Geometry: final body of the model. Coordinates: model frame, mm. Face numbers are marked on the shaded views. Coordinates: 2 decimals unless noted, no trailing zeros. Put each result on its own line as item: value.
```python
from build123d import *

# Parameters (mm, degrees)
CROQUIS1_R                  = 16.5
CROQUIS1_R_2                = 3.75
CROQUIS1_R_3                = 1.5
SALIENTE_EXTRUIR1_DEPTH     = 5
CROQUIS2_R                  = 5.5
CORTAR_EXTRUIR1_DEPTH       = 2
CORTAR_EXTRUIR2_START       = -5
CROQUIS4_R                  = 3
CORTAR_EXTRUIR2_DEPTH       = 2.5
CROQUIS6_R                  = 1.5
SALIENTE_EXTRUIR3_DEPTH     = 5
SALIENTE_EXTRUIR4_START     = -5
SALIENTE_EXTRUIR4_DEPTH     = 5
CORTAR_EXTRUIR3_START       = -5
CORTAR_EXTRUIR3_OUTLINE_R   = 1.5
CORTAR_EXTRUIR3_OUTLINE_R_2 = 3.75
CORTAR_EXTRUIR3_DEPTH       = 5


# Read off the part's stored shape, not the designer's step: Saliente-Extruir4, Cortar-Extruir3
with BuildPart() as part:
    # Croquis1 → Saliente-Extruir1 (new body)
    with BuildSketch(Plane(origin=(0, 0, 0), x_dir=(1, 0, 0), z_dir=(0, 1, 0))):
        with Locations(Location((0, 0, 0), (0, 0, 270))):
            Circle(CROQUIS1_R)
        with Locations(Location((0, 0, 0), (0, 0, 270))):
            Circle(CROQUIS1_R_2, mode=Mode.SUBTRACT)
        with Locations(Location((10, 0, 0), (0, 0, 270))):
            Circle(CROQUIS1_R_3, mode=Mode.SUBTRACT)
        with Locations(Location((0, -10, 0), (0, 0, 270))):
            Circle(CROQUIS1_R_3, mode=Mode.SUBTRACT)
        with Locations(Location((-10, 0, 0), (0, 0, 270))):
            Circle(CROQUIS1_R_3, mode=Mode.SUBTRACT)
        with Locations(Location((0, 10, 0), (0, 0, 270))):
            Circle(CROQUIS1_R_3, mode=Mode.SUBTRACT)
    extrude(amount=SALIENTE_EXTRUIR1_DEPTH)

    # Croquis2 → Cortar-Extruir1 (cut)
    with BuildSketch(Plane(origin=(0, 5, 0), x_dir=(1, 0, 0), z_dir=(0, 1, 0))):
        with Locations(Location((0, 0, 0), (0, 0, 270))):
            Circle(CROQUIS2_R)
    extrude(amount=-CORTAR_EXTRUIR1_DEPTH, mode=Mode.SUBTRACT)

    # Croquis4 → Cortar-Extruir2 (cut)
    with BuildSketch(Plane(origin=(0, 5, 0), x_dir=(1, 0, 0), z_dir=(0, 1, 0)).offset(CORTAR_EXTRUIR2_START)):
        with Locations(Location((10, 0, 0), (0, 0, 270))):
            Circle(CROQUIS4_R)
        with Locations(Location((-10, 0, 0), (0, 0, 270))):
            Circle(CROQUIS4_R)
        with Locations(Location((0, 10, 0), (0, 0, 270))):
            Circle(CROQUIS4_R)
    extrude(amount=CORTAR_EXTRUIR2_DEPTH, mode=Mode.SUBTRACT)

    # Croquis6 → Saliente-Extruir3 (add)
    with BuildSketch(Plane(origin=(0, 5, 0), x_dir=(1, 0, 0), z_dir=(0, 1, 0))):
        with BuildLine():
            Line((-16.499999253, -0.004966275), (0, -15.162135144))
            Line((0, -15.162135144), (16.499999253, -0.004966275))
            add(Edge.make_bspline(
                [(16.499999253, -0.004966275), (14.789720677, -16.601874141), (14.779811161, -16.438973164), (14.200732618, -20.551745369), (13.635520661, -22.485602375), (15.733267293, -30.419610193), (11.37636727, -34.073606125), (1.56418736, -36.497980996), (2.416281914, -27.975905143), (1.888822796, -23.5), (0, -23.5)],
                knots=[0, 0, 0, 0, 0.196162037, 0.24321543, 0.470533934, 0.661030556, 0.708413553, 0.918147195, 0.949927511, 1, 1, 1, 1], degree=3))
            add(Edge.make_bspline(
                [(-16.499999253, -0.004966275), (-14.789720677, -16.601874141), (-14.779811161, -16.438973164), (-14.200732618, -20.551745369), (-13.635520661, -22.485602375), (-15.733267293, -30.419610193), (-11.37636727, -34.073606125), (-1.56418736, -36.497980996), (-2.416281914, -27.975905143), (-1.888822796, -23.5), (0, -23.5)],
                knots=[0, 0, 0, 0, 0.196162037, 0.24321543, 0.470533934, 0.661030556, 0.708413553, 0.918147195, 0.949927511, 1, 1, 1, 1], degree=3))
        make_face()
        with Locations(Location((-8, -30.5, 0), (0, 0, 270))):
            Circle(CROQUIS6_R, mode=Mode.SUBTRACT)
        with Locations(Location((8, -30.5, 0), (0, 0, 90))):
            Circle(CROQUIS6_R, mode=Mode.SUBTRACT)
    extrude(amount=-SALIENTE_EXTRUIR3_DEPTH)

    # Saliente-Extruir4 outline → Saliente-Extruir4 (add)
    with BuildSketch(Plane(origin=(0, 5, 0), x_dir=(1, 0, 0), z_dir=(0, 1, 0)).offset(SALIENTE_EXTRUIR4_START)):
        with BuildLine():
            add(Edge.make_bspline(
                [(14.291966708, -31.373017759), (14.340514678, -31.295086469), (14.385698727, -31.215084368), (14.427688557, -31.133168853)],
                knots=[0.343293779, 0.343293779, 0.343293779, 0.343293779, 0.350896071, 0.350896071, 0.350896071, 0.350896071], degree=3))
            add(Edge.make_bspline(
                [(14.291966708, -31.373017759), (14.349575443, -31.290166182), (14.395146457, -31.209972546), (14.427688557, -31.133168853)],
                knots=[0.96489404, 0.96489404, 0.96489404, 0.96489404, 1, 1, 1, 1], degree=3))
        make_face()
        with BuildLine():
            add(Edge.make_bspline(
                [(-14.427688557, -31.133168853), (-14.395146457, -31.209972546), (-14.349575443, -31.290166182), (-14.291966708, -31.373017759)],
                knots=[0, 0, 0, 0, 0.03510596, 0.03510596, 0.03510596, 0.03510596], degree=3))
            add(Edge.make_bspline(
                [(-14.427688557, -31.133168853), (-14.385698727, -31.215084368), (-14.340514678, -31.295086469), (-14.291966708, -31.373017759)],
                knots=[0.649103929, 0.649103929, 0.649103929, 0.649103929, 0.656706221, 0.656706221, 0.656706221, 0.656706221], degree=3))
        make_face()
        with BuildLine():
            add(Edge.make_bspline(
                [(0, -33.607159893), (1.397517326, -33.429434313), (2.728240909, -33.755145964), (4.099311118, -34.046838013)],
                knots=[0, 0, 0, 0, 0.263268598, 0.263268598, 0.263268598, 0.263268598], degree=3))
            add(Edge.make_bspline(
                [(0, -23.5), (1.888822796, -23.5), (2.416281914, -27.975905143), (1.994660589, -32.192677678), (3.074818283, -33.563655557), (4.099311118, -34.046838013)],
                knots=[0, 0, 0, 0, 0.050072489, 0.081852805, 0.144278664, 0.144278664, 0.144278664, 0.144278664], degree=3))
            add(Edge.make_bspline(
                [(-4.099311115, -34.046838012), (-3.074818281, -33.563655555), (-1.994660589, -32.192677676), (-2.416281914, -27.975905143), (-1.888822796, -23.5), (0, -23.5)],
                knots=[0.855721336, 0.855721336, 0.855721336, 0.855721336, 0.918147195, 0.949927511, 1, 1, 1, 1], degree=3))
            add(Edge.make_bspline(
                [(-4.099311115, -34.046838012), (-2.728240907, -33.755145963), (-1.397517325, -33.429434314), (0, -33.607159893)],
                knots=[0.736731402, 0.736731402, 0.736731402, 0.736731402, 1, 1, 1, 1], degree=3))
        make_face()
    extrude(amount=SALIENTE_EXTRUIR4_DEPTH)

    # Cortar-Extruir3 outline → Cortar-Extruir3 (cut)
    with BuildSketch(Plane(origin=(0, 5, 0), x_dir=(1, 0, 0), z_dir=(0, 1, 0)).offset(CORTAR_EXTRUIR3_START)):
        with BuildLine():
            add(Edge.make_bspline(
                [(-5, -5.704095984), (-6.82751306, -5.704095984), (-11.278769384, -9.499460435), (-13.360021763, -18.603666683), (-13.970897338, -21.999566183)],
                knots=[0, 0, 0, 0, 0.255170628, 0.749384094, 0.749384094, 0.749384094, 0.749384094], degree=3))
            Line((-5, -5.704095984), (5, -5.704095984))
            add(Edge.make_bspline(
                [(5, -5.704095984), (10.679811422, -5.704095984), (13.347569143, -18.187313933), (14.115183744, -22.835331636)],
                knots=[0, 0, 0, 0, 0.793056467, 0.793056467, 0.793056467, 0.793056467], degree=3))
            add(Edge.make_bspline(
                [(14.115183744, -22.835331636), (13.982038213, -21.263217458), (14.258823228, -20.139170168), (14.762278608, -16.563494089), (14.787566831, -16.590643141), (16.153585525, -3.36328332)],
                knots=[0.576667959, 0.576667959, 0.576667959, 0.576667959, 0.75678457, 0.803837963, 0.985753813, 0.985753813, 0.985753813, 0.985753813], degree=3))
            ThreePointArc((16.153585525, -3.36328332), (0, 16.5), (-16.153585525, -3.36328332))
            add(Edge.make_bspline(
                [(-16.153585525, -3.36328332), (-14.787566831, -16.590643141), (-14.762278608, -16.563494089), (-14.261753936, -20.118355485), (-13.987841454, -21.239556576), (-14.110086789, -22.773329956)],
                knots=[0.014246187, 0.014246187, 0.014246187, 0.014246187, 0.196162037, 0.24321543, 0.420950675, 0.420950675, 0.420950675, 0.420950675], degree=3))
            Line((-14.110086789, -22.773329956), (-13.970897338, -21.999566183))
        make_face()
        with Locations((-10, 0)):
            Circle(CORTAR_EXTRUIR3_OUTLINE_R, mode=Mode.SUBTRACT)
        Circle(CORTAR_EXTRUIR3_OUTLINE_R_2, mode=Mode.SUBTRACT)
        with Locations((10, 0)):
            Circle(CORTAR_EXTRUIR3_OUTLINE_R, mode=Mode.SUBTRACT)
        with Locations((0, 10)):
            Circle(CORTAR_EXTRUIR3_OUTLINE_R, mode=Mode.SUBTRACT)
    extrude(amount=CORTAR_EXTRUIR3_DEPTH, mode=Mode.SUBTRACT)


solid = part.part
```
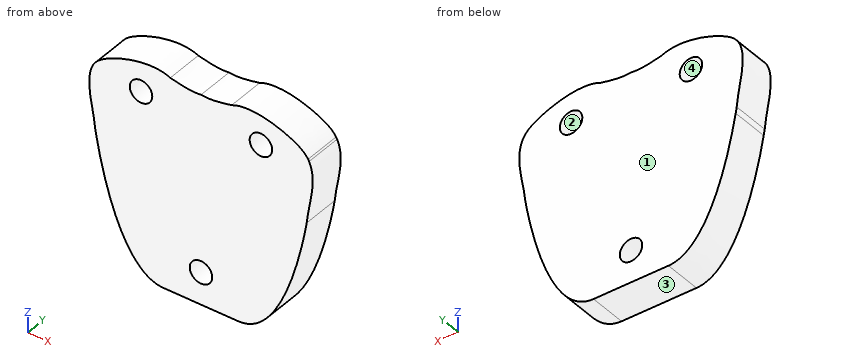
1. Section query A-A (y = 2.25). Count the separate pieces of the cut face and the enclosed holes in it, then the cut area to 3 significant figures.
Answer below:
separate pieces: 1
enclosed holes: 3
area: 691 mm²
2. Ray query, probe 1 along X at (y, z) = (3.65, 30.5); probe 2 along Z at (x, y) = (9, 3.6); probe 3 along Z at (x, y) = (8, 2.15). Return the intervals inside material, ascending. Write a range as from..to.
Answer below:
probe 1: x = -14.68..-9.5, -6.5..6.5, 9.5..14.68
probe 2: z = 8.08..29.38, 31.62..34.18
probe 3: z = 6.99..29, 32..34.37
3. Mould query, pull axis Z, two halves, no side actions, for the marked faces 1, 2, 3 and 4. Classes: +Z half, -Z half, draft (parallel to the pull), parting line (faces both ways), or undercut.
Answer below:
face 1: draft
face 2: undercut
face 3: -Z half
face 4: undercut
4. Pin query (flat end, axial travel): pin 1 Ø5 at (x, z) = (-8, 30.5) entering from -Y; pin 2 Ø2 at (x, y) = (11.5, 4) entering from -Z. Return the tip coordinate at first contact, or that it passes through.
Answer below:
pin 1: stops at y = 0
pin 2: stops at z = 10.51
